Here's how the part is built. I have some questions about the finished solid (model axes, mm). Face numbers are marked on the shaded views. A direction names the side the tool comes from. Coordinates: 2 decimals unless noted, no trailing zeros. Write each loop counter-clockwise with the first axis right and the second up, starting at its lowest first coordinate (ties: lowest second). Pieces come first, ordered by that corner, then holes.
Item 1: I want a section at B-B (x = 36.5). Please give me the cut outline in (y, z).
Item 2: I want a section at C-C (z = -21). Please give me the cut outline in (x, y), and give its area (3 significant figures).
Item 3: Please list where these lines run through material, in increasing order: line 1 (X direction, y = 1.55, z = -36.5); line 2 (X direction, y = 1, z = -21); line 3 (Y direction, x = -0.7, z = -21).
Item 4: I want a section at A-A (x = 1). Please give me the cut outline in (y, z), and give its area (3 significant figures).
Item 5: I'm going to push flat-ended pins straight in: P1, Ø1.8, axis at x = 36.5, z = -36.5, coming from the +Y side; P2, Ø4, axis at y = -40, z = -21.5, coming from the +X side; P3, Ø12.5, axis at x = 16, z = -24, coming from the -Y side; P4, Ø18, axis at y = -11.5, z = -21.5, coming from the +X side. Where does each tip first touch, or does it pass through?
Item 6: For the marked faces 1 and 2, which set-ups out of +Z, -Z, +X, -X, +Y, -Y let a thin tool reach every point of the face, with its end or its side?
Item 7: I want a section at D-D (x = 21). Please give me the cut outline in (y, z), and give its area (3 significant figures).
Item 8: If we mould it in two halves opening along Y, with no side actions, what happens to the marked faces 3, 4 and 5? For each: pulls with the +Y half, pulls with the -Y half, needs draft (parallel to the pull), parting line crosses it, or undercut.
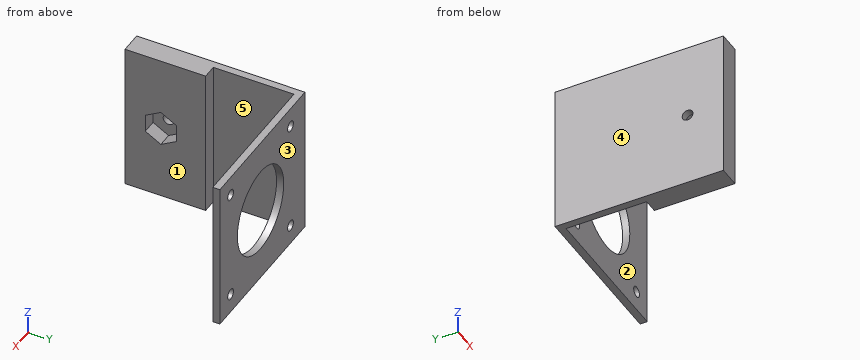
from build123d import *

# Parameters (mm, degrees)
SKETCH_1_W          = 42
SKETCH_1_H          = 42
EXTRUDE_1_DEPTH     = 2
SKETCH_2_R          = 12
SKETCH_2_R_2        = 1.5
CUT_EXTRUDE_1_DEPTH = 2
SKETCH_3_W          = 42
SKETCH_3_H          = 2
EXTRUDE_3_DEPTH     = 2
SKETCH_4_W          = 2
SKETCH_4_H          = 42
EXTRUDE_4_DEPTH     = 45
EXTRUDE_5_DEPTH     = 4
CUT_EXTRUDE_2_DEPTH = 4
CUT_EXTRUDE_3_DEPTH = 4


with BuildPart() as part:
    # 草图1 → 凸台-拉伸1 (new body)
    with BuildSketch(Plane(origin=(0, 0, 0), x_dir=(1, 0, 0), z_dir=(0, 1, 0))):
        with Locations((21, 21)):
            Rectangle(SKETCH_1_W, SKETCH_1_H)
    extrude(amount=EXTRUDE_1_DEPTH)

    # 草图2 → 切除-拉伸1 (cut)
    with BuildSketch(Plane(origin=(0, 2, 0), x_dir=(1, 0, 0), z_dir=(0, 1, 0))):
        with Locations(Location((21, 21, 0), (0, 0, 270))):
            Circle(SKETCH_2_R)
        with Locations(Location((36.5, 36.5, 0), (0, 0, 270))):
            Circle(SKETCH_2_R_2)
        with Locations(Location((36.5, 5.5, 0), (0, 0, 270))):
            Circle(SKETCH_2_R_2)
        with Locations(Location((5.5, 5.5, 0), (0, 0, 270))):
            Circle(SKETCH_2_R_2)
        with Locations(Location((5.5, 36.5, 0), (0, 0, 270))):
            Circle(SKETCH_2_R_2)
    extrude(amount=-CUT_EXTRUDE_1_DEPTH, mode=Mode.SUBTRACT)

    # 草图3 → 凸台-拉伸3 (add)
    with BuildSketch(Plane.ZY):
        with Locations((-21, 1)):
            Rectangle(SKETCH_3_W, SKETCH_3_H)
    extrude(amount=EXTRUDE_3_DEPTH)

    # 草图4 → 凸台-拉伸4 (add)
    with BuildSketch(Plane.XZ):
        with Locations((-1, -21)):
            Rectangle(SKETCH_4_W, SKETCH_4_H)
    extrude(amount=EXTRUDE_4_DEPTH)

    # 草图5 → 凸台-拉伸5 (add)
    with BuildSketch(Plane(origin=(0, 0, 0), x_dir=(0, 0, -1), z_dir=(1, 0, 0))):
        Polygon((0, -22.5), (0, -45), (42, -45), (42, -22.5), (21, -22.5), align=None)
    extrude(amount=EXTRUDE_5_DEPTH)

    # 草图6 → 切除-拉伸2 (cut)
    with BuildSketch(Plane(origin=(4, 0, 0), x_dir=(0, 0, -1), z_dir=(1, 0, 0))):
        Polygon((26, -35), (23.5, -30.669872981), (18.5, -30.669872981), (16, -35), (18.5, -39.330127019), (23.5, -39.330127019), align=None)
    extrude(amount=-CUT_EXTRUDE_2_DEPTH, mode=Mode.SUBTRACT)

    # 草图7 → 切除-拉伸3 (cut)
    with BuildSketch(Plane(origin=(0, 0, 0), x_dir=(0, 0, -1), z_dir=(1, 0, 0))):
        with BuildLine():
            ThreePointArc((22.5, -35), (21, -33.5), (19.5, -35))
            Line((19.5, -35), (22.5, -35))
        make_face()
        with BuildLine():
            Line((22.5, -35), (19.5, -35))
            ThreePointArc((19.5, -35), (21, -36.5), (22.5, -35))
        make_face()
    extrude(amount=-CUT_EXTRUDE_3_DEPTH, mode=Mode.SUBTRACT)


solid = part.part
Answer:
1. outline: (0, -42) - (2, -42) - (2, -38) - (0, -38) - close; (0, -35) - (2, -35) - (2, -7) - (0, -7) - close; (0, -4) - (2, -4) - (2, 0) - (0, 0) - close
2. outline: (-2, -45) - (4, -45) - (4, -39.33) - (0, -39.33) - (0, -36.5) - (-2, -36.5) - close; (-2, -33.5) - (0, -33.5) - (0, -30.67) - (4, -30.67) - (4, -22.5) - (0, -22.5) - (0, 0) - (9, 0) - (9, 2) - (-2, 2) - close; (33, 0) - (42, 0) - (42, 2) - (33, 2) - close
2. area: 179 mm2
3. line 1: x = -2 to 4, 7 to 35, 38 to 42
3. line 2: x = -2 to 9, 33 to 42
3. line 3: y = -45 to -36.5, -33.5 to 2
4. outline: (-45, -42) - (-22.5, -42) - (-22.5, 0) - (-45, 0) - close; (0, -42) - (2, -42) - (2, 0) - (0, 0) - close; hole (-39.33, -23.5) - (-35, -26) - (-30.67, -23.5) - (-30.67, -18.5) - (-35, -16) - (-39.33, -18.5) - close
4. area: 964 mm2
5. P1: passes through
5. P2: stops at x = 4
5. P3: stops at y = 0
5. P4: stops at x = 0
6. face 1: +Z, -Z, +X, -Y
6. face 2: +Z, -Z, +X
7. outline: (0, -42) - (2, -42) - (2, -33) - (0, -33) - close; (0, -9) - (2, -9) - (2, 0) - (0, 0) - close
7. area: 36.0 mm2
8. face 3: pulls with the +Y half
8. face 4: needs draft
8. face 5: undercut
